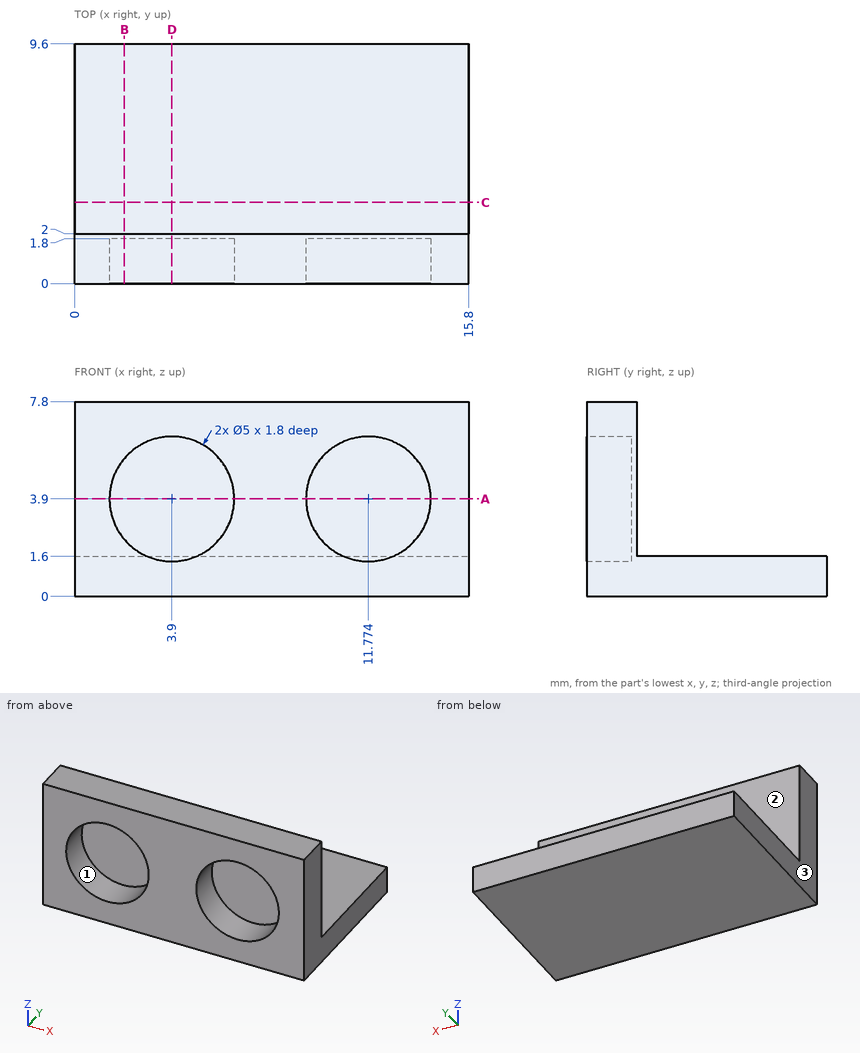
Job drawing, mm, ordinate dimensions from the low corner. One solid piece. A direction names the side the tool comes from. Give positions to 0.01 mm unless a question says otherwise; leave off trailing zeros. Write each loop counter-clockwise with the first axis right and the second up, starting at its lowest first coordinate (ties: lowest second). Pieces come first, ordered by that corner, then holes. Notation, with made-up numbers: (16, 49.25) -> (39, 49.25) arc R21 cw to (39, 56.25) -> close; hole circle Ø10 at (16, 40). An arc over 180 degrees is marked (long way). Return JSON: item names as keys, results as strings.
Item 1: Band-saw the part on C-C (y = 3.25). List the corners of the cut face in (x, z), then the cut area to 3 significant figures.
Answer below:
{"outline": "(0, 0) -> (15.8, 0) -> (15.8, 1.6) -> (0, 1.6) -> close", "area": "25.3 mm2"}
Item 2: Band-saw the part on A-A (z = 3.9). List the corners of the cut face in (x, y), then the cut area to 3 significant figures.
Answer below:
{"outline": "(0, 0) -> (1.4, 0) -> (1.4, 1.8) -> (6.4, 1.8) -> (6.4, 0) -> (9.27, 0) -> (9.27, 1.8) -> (14.27, 1.8) -> (14.27, 0) -> (15.8, 0) -> (15.8, 2) -> (0, 2) -> close", "area": "13.6 mm2"}
Item 3: Drop flat-ended pins along their axis: pin 1 (2.5 mm diameter, centred on x = 9, y = 7, fed in from +Z); pin 2 (4 mm diameter, centred on x = 4.5, z = 5, fed in from +Y); pin 3 (1.5 mm diameter, centred on x = 4, z = 4.5, fed in from -Y). Give the stop position or say it passes through.
Answer below:
{"pin 1": "stops at z = 1.6", "pin 2": "stops at y = 2", "pin 3": "stops at y = 1.8"}
Item 4: Band-saw the part on D-D (x = 3.9). List the corners of the cut face in (y, z), then the cut area to 3 significant figures.
Answer below:
{"outline": "(0, 0) -> (9.6, 0) -> (9.6, 1.6) -> (2, 1.6) -> (2, 7.8) -> (0, 7.8) -> (0, 6.4) -> (1.8, 6.4) -> (1.8, 1.4) -> (0, 1.4) -> close", "area": "18.8 mm2"}
Item 5: Drill centre lines: probe 1 along X at (y, z) = (1.2, 3.9); probe 2 along Z at (x, y) = (15, 9.25); probe 3 along Y at (x, z) = (7.75, 4.25). Where is each one in solid material? Low to high.
Answer below:
{"probe 1": "x = 0 to 1.4, 6.4 to 9.27, 14.27 to 15.8", "probe 2": "z = 0 to 1.6", "probe 3": "y = 0 to 2"}
Item 6: Band-saw the part on B-B (x = 2). List the corners of the cut face in (y, z).
Answer below:
{"outline": "(0, 0) -> (9.6, 0) -> (9.6, 1.6) -> (2, 1.6) -> (2, 7.8) -> (0, 7.8) -> (0, 5.52) -> (1.8, 5.52) -> (1.8, 2.28) -> (0, 2.28) -> close"}
Item 7: Tool access for the marked faces 1, 2 and 3: list every direction of +Z, -Z, +X, -X, +Y, -Y with a clear straight run to the whole face (end or side of a thin tool).
Answer below:
{"face 1": "-Y", "face 2": "+Z, +X, -X, +Y", "face 3": "+Z, -Z, -X, +Y, -Y"}
